Model file for the job. Use its own axes, mm. Face numbers are marked on the shaded views. A direction names the side the tool comes from. Round coordinates to 2 decimals unless told otherwise and drop trailing zeros. Loops run counter-clockwise (first coordinate to the right, second up) from the corner with the lowest first, then second, coordinate; pieces in that order, holes last.
from build123d import *

# Parameters (mm, degrees)
SALIENTE_EXTRUIR1_DEPTH = 70
VACIADO1_T              = -2
CORTAR_EXTRUIR1_REACH   = 135.884
CROQUIS4_W              = 22.5
CROQUIS4_H              = 12.2
REDONDEO1_R             = 5
CHAFL_N1_SIZE           = 0.12
CHAFL_N2_SIZE           = 0.2


with BuildPart() as part:
    # Croquis1 → Saliente-Extruir1 (new body)
    with BuildSketch(Plane.XY):
        Polygon((30, 50), (-30, 50), (-55, 25), (-55, -25), (-30, -50), (30, -50), (55, -25), (55, 25), align=None)
    extrude(amount=SALIENTE_EXTRUIR1_DEPTH)

    # Vaciado1
    vaciado1_openings = [part.faces().sort_by_distance(p)[0] for p in [
        (0, 0, 70),
    ]]
    offset(amount=VACIADO1_T, openings=vaciado1_openings, kind=Kind.INTERSECTION)

    # Croquis4 → Cortar-Extruir1 (cut, up to next)
    with BuildSketch(Plane.XZ.offset(50), mode=Mode.PRIVATE) as cortar_extruir1_sk1:
        with Locations((-5.15, 22)):
            Rectangle(CROQUIS4_W, CROQUIS4_H)
    cortar_extruir1_tool1 = extrude(cortar_extruir1_sk1.sketch, amount=-CORTAR_EXTRUIR1_REACH, mode=Mode.PRIVATE) & part.part
    cortar_extruir1 = cortar_extruir1_tool1.solids().sort_by_distance((-5.15, -50, 22))[0]
    add(cortar_extruir1, mode=Mode.SUBTRACT)

    # Simetría1: Cortar-Extruir1 across plane
    add(cortar_extruir1.mirror(Plane.ZX), mode=Mode.SUBTRACT)

    # Redondeo1
    redondeo1_edges = [part.edges().sort_by_distance(p)[0] for p in [
        (41.085786438, -36.085786438, 2),
        (53, 0, 2),
        (41.085786438, 36.085786438, 2),
        (0, 48, 2),
        (-41.085786438, 36.085786438, 2),
        (-53, 0, 2),
        (-41.085786438, -36.085786438, 2),
        (0, -48, 2),
    ]]
    fillet(redondeo1_edges, radius=REDONDEO1_R)

    # Chaflán1
    chafl_n1_edges = [part.edges().sort_by_distance(p)[0] for p in [
        (0, 50, 0),
        (42.5, 37.5, 0),
        (55, 0, 0),
        (42.5, -37.5, 0),
        (0, -50, 0),
        (-42.5, -37.5, 0),
        (-55, 0, 0),
        (-42.5, 37.5, 0),
    ]]
    chamfer(chafl_n1_edges, length=CHAFL_N1_SIZE)

    # Chaflán2
    chafl_n2_edges = [part.edges().sort_by_distance(p)[0] for p in [
        (-5.15, -48, 15.9),
        (6.1, -48, 22),
        (-5.15, -48, 28.1),
        (-16.4, -48, 22),
        (-5.15, 48, 28.1),
        (-16.4, 48, 22),
        (-5.15, 48, 15.9),
        (6.1, 48, 22),
    ]]
    chamfer(chafl_n2_edges, length=CHAFL_N2_SIZE)


solid = part.part
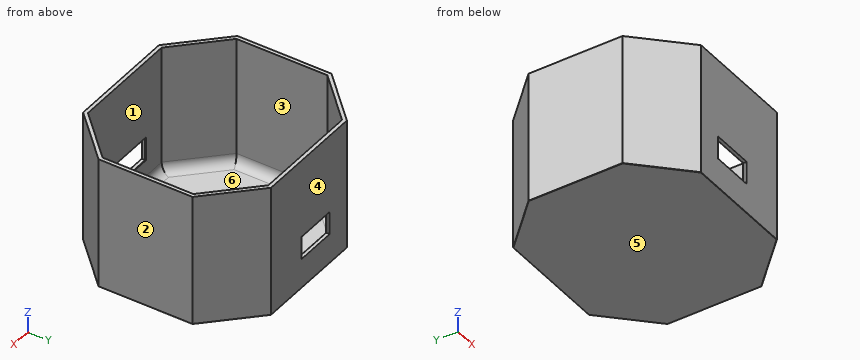
Q1. Slice it at D-D on x = 15.5. Give the cut face in (y, z), plus the area to 3 significant figures.
Q2. Flat gauge pins, fed straight in: P1, Ø1.5, axis at y = 34, z = 24, coming from the -X side; P2, Ø0.5, axis at y = -49, z = 25, coming from the +X side; P3, Ø3, axis at x = -29, y = -12, coming from the +Z side. Where does each tip first touch, or does it go through?
Q3. Slice it at A-A on x = -14.5. Give the cut face in (y, z).
Q4. Slice it at C-C on y = 12. Give the cut face in (x, z).
Q5. Tool access for the marked faces 1 and 2: list every direction of +Z, -Z, +X, -X, +Y, -Y with a clear straight run to the whole face (end or side of a thin tool).
Q6. Pull direction Y, two halves, no side cores. Call the marked faces 3, 4, 5 and 6: pulls with the +Y half, pulls with the -Y half, needs draft (parallel to the pull), parting line crosses it, or undercut.
Q7. Probe line 1 (Y direction, x = -6, z = 59.5); line 2 (X direction, y = -21, z = 18); line 3 (Z direction, x = -7.5, y = 40.5). List the from-to ranges inside material, lowest first.
Q8. Slice it at B-B on z = 57.5. Give the cut face in (x, y), plus the area to 3 significant figures.
Reply:
1. outline: (-50, 0.12) - (-49.88, 0) - (49.88, 0) - (50, 0.12) - (50, 70) - (48, 70) - (48, 7) arc R5 cw to (43, 2) - (-43, 2) arc R5 cw to (-48, 7) - (-48, 70) - (-50, 70) - close
1. area: 483 mm2
2. P1: stops at x = -46.75
2. P2: stops at x = 31.25
2. P3: stops at z = 2
3. outline: (-50, 0.12) - (-49.88, 0) - (49.88, 0) - (50, 0.12) - (50, 15.9) - (48.2, 15.9) - (48, 15.7) - (48, 7) arc R5 cw to (43, 2) - (-43, 2) arc R5 cw to (-48, 7) - (-48, 15.7) - (-48.2, 15.9) - (-50, 15.9) - close; (-50, 28.1) - (-48.2, 28.1) - (-48, 28.3) - (-48, 70) - (-50, 70) - close; (48, 28.3) - (48.2, 28.1) - (50, 28.1) - (50, 70) - (48, 70) - close
4. outline: (-55, 0.12) - (-54.88, 0) - (54.88, 0) - (55, 0.12) - (55, 70) - (53, 70) - (53, 7) arc R5 cw to (48, 2) - (-48, 2) arc R5 cw to (-53, 7) - (-53, 70) - (-55, 70) - close
5. face 1: +Z
5. face 2: +Z, -Z, +X, +Y, -Y
6. face 3: undercut
6. face 4: pulls with the +Y half
6. face 5: needs draft
6. face 6: undercut
7. line 1: y = -50 to -48, 48 to 50
7. line 2: x = -55 to -53, 53 to 55
7. line 3: z = 0 to 2
8. outline: (-55, -25) - (-30, -50) - (30, -50) - (55, -25) - (55, 25) - (30, 50) - (-30, 50) - (-55, 25) - close; hole (-53, -24.17) - (-29.17, -48) - (29.17, -48) - (53, -24.17) - (53, 24.17) - (29.17, 48) - (-29.17, 48) - (-53, 24.17) - close
8. area: 710 mm2
